from build123d import *

# Parameters (mm, degrees)
F0_W     = 38.1
F0_H     = 44.45
F1_DEPTH = 25.4
F3_DEPTH = 25.401
F5_DEPTH = 25.401
F6_W     = 12.7
F6_H     = 6.35
F7_DEPTH = 25.401


with BuildPart() as f1:
    # F0 (on Front) → F1 (new body)
    with BuildSketch(Plane.XZ):
        with Locations((-1.822717, 23.700186)):
            Rectangle(F0_W, F0_H)
    extrude(amount=F1_DEPTH)

    # F2 (on face) → F3 (cut, through all)
    with BuildSketch(Plane.XZ.offset(25.4)):
        Polygon((17.227283, 45.925186), (4.527283, 45.925186), (17.227283, 1.475186), align=None)
    extrude(amount=-F3_DEPTH, mode=Mode.SUBTRACT)

    # F4 (on face) → F5 (cut, through all)
    with BuildSketch(Plane.XZ.offset(25.4)):
        Polygon((-20.872717, 1.475186), (-8.172717, 45.925186), (-20.872717, 45.925186), align=None)
    extrude(amount=-F5_DEPTH, mode=Mode.SUBTRACT)

    # F6 (on face) → F7 (cut, through all)
    with BuildSketch(Plane.XZ.offset(25.4)):
        with Locations((-1.822717, 4.650186)):
            Rectangle(F6_W, F6_H)
    extrude(amount=-F7_DEPTH, mode=Mode.SUBTRACT)


solid = f1.part
Read the model definition and answer for the solid it produces. Units are mm, in the model's axes. A direction names the side the tool comes from. Give positions to 0.01 mm unless a question says otherwise; leave off trailing zeros. Loops run counter-clockwise (first coordinate to the right, second up) from the corner with the lowest first, then second, coordinate; pieces in that order, holes last. Notation, with made-up numbers: (24, 52) -> (47, 52) arc R26 cw to (47, 89) -> close; hole circle Ø4 at (-14, 18). An arc over 180 degrees is marked (long way). Use a Markdown table: item, result.
Q1. A tool of negligible diameter and unlimited length cuts with its end or side. For faces 5 (the face through (-8.173, -13, 5)), 6 (the face through (-2, 0, 19)), from which of +Z, -Z, +X, -X, +Y, -Y can it reach the whole face along a straight path? Write none if from no direction.
Solved:
| item | result |
|---|---|
| face 5 | -Z, +Y, -Y |
| face 6 | +Z, -Z, +X, -X, +Y |
Q2. Section C-C, the plane z = 17 is taken. Determine the outline of the cut face in (x, y).
Solved:
| item | result |
|---|---|
| outline | (-16.44, -25.4) -> (12.79, -25.4) -> (12.79, 0) -> (-16.44, 0) -> close |
Q3. Section B-B, the plane x = -2.5 is taken. Determine the outline of the cut face in (y, z), then the cut area to 3 significant figures.
Solved:
| item | result |
|---|---|
| outline | (-25.4, 7.83) -> (0, 7.83) -> (0, 45.93) -> (-25.4, 45.93) -> close |
| area | 968 mm^2 |
Q4. Section A-A, the plane y = -15 is taken. Determine the outline of the cut face in (x, z).
Solved:
| item | result |
|---|---|
| outline | (-20.87, 1.48) -> (-8.17, 1.48) -> (-8.17, 7.83) -> (4.53, 7.83) -> (4.53, 1.48) -> (17.23, 1.48) -> (4.53, 45.93) -> (-8.17, 45.93) -> close |
Q5. Find the intervals of material crossed by line 1 along Z through (x, y) = (-5, -8.5); line 2 along X through (y, z) = (-23.75, 4); line 3 along X through (y, z) = (-15.25, 24), in increasing order.
Solved:
| item | result |
|---|---|
| line 1 | z = 7.83 to 45.93 |
| line 2 | x = -20.15 to -8.17, 4.53 to 16.51 |
| line 3 | x = -14.44 to 10.79 |
Q6. Each of these flat-tipped pins is pushed along its axis until it touches: pin 1 (1.5 mm diameter, centred on y = -2.5, z = 33, fed in from -X); pin 2 (3 mm diameter, centred on y = -16, z = 4.5, fed in from -X); pin 3 (2 mm diameter, centred on y = -20.5, z = 11, fed in from +X); pin 4 (8 mm diameter, centred on x = 4.5, z = 11.5, fed in from +Y). Where does it stop, or does it pass through?
Solved:
| item | result |
|---|---|
| pin 1 | stops at x = -12.08 |
| pin 2 | stops at x = -20.44 |
| pin 3 | stops at x = 14.79 |
| pin 4 | stops at y = 0 |
Q7. Determine the mould class of faces 1 (the face through (-2, -13, 7.825)), 2 (the face through (-2, -13, 45.925)), 3 (the face through (4.527, -13, 5)), 4 (the face through (10.79, -12.88, 24.01)) for opening direction X: pulls with the +X half, pulls with the -X half, needs draft (parallel to the pull), parting line crosses it, or undercut.
Solved:
| item | result |
|---|---|
| face 1 | undercut |
| face 2 | needs draft |
| face 3 | undercut |
| face 4 | pulls with the +X half |
